Verification items for the finished model (mm, model axes). Coordinates: 2 decimals unless noted, no trailing zeros. Loops run counter-clockwise (first coordinate to the right, second up) from the corner with the lowest first, then second, coordinate; pieces in that order, holes last.
Q1. Sectioned sample at C-C (x = -37.5). Enter the section's corners in (y, z), then the cut area to 3 significant figures.
Q2. Go/stop test with flat-tipped pins: P1, Ø1.9, axis at y = -36, z = 3.5, coming from the -X side; P2, Ø5.5, axis at x = -37.5, y = 0, coming from the +Z side; P3, Ø1.5, axis at x = -16, z = 1.5, coming from the +Y side; P4, Ø3, axis at x = 35, z = 3.5, coming from the -Y side. Record where each tip stops, or that it passes through.
Q3. Sectioned sample at B-B (y = 0). Enter the section's corners in (x, z), then the cut area to 3 significant figures.
Q4. Mould release check, pull along X, two halves, no side actions. Record for faces 1 (the face through (1.47, 49.98, 3.13)), 2 (the face through (-13.675, -34.628, 3.272)), 3 (the face through (-35.302, 0.097, 2.007)): +X half, -X half, draft (parallel to the pull), parting line (faces both ways), or undercut.
Q5. Sectioned sample at D-D (x = -15). Enter the section's corners in (y, z) (3 decimals).
Q6. Material ranges on probe 1 along X at (y, z) = (-20, 1.7); probe 2 along Y at (x, z) = (-5.5, 2); probe 3 along Y at (x, z) = (-1.5, 5.75), recorded low to high.
Q7. Sectioned sample at A-A (x = 0). Enter the section's corners in (y, z).
```python
from build123d import *

# Parameters (mm, degrees)
F0_R           = 50
F1_DEPTH       = 6.35
F3_D           = 4.4
F3_CSINK_D     = 8.96
F3_CSINK_ANGLE = 90
F4_R           = 8
F5_DEPTH       = 8
F7_DEPTH       = 25
F9_R           = 5
F10_D          = 4.4
F11_R          = 7.5
F12_DEPTH      = 25


# Not quite as in the source:
# - a feature names something its author has since deleted; it is built from what else it names


with BuildPart() as f1:
    # F0 (on Top) → F1 (new body)
    with BuildSketch(Plane.XY):
        Circle(F0_R)
    extrude(amount=F1_DEPTH)

    # F3 (through all)
    with Locations(Plane.XY.offset(6.35)):
        with Locations((-37.5, 20), (-37.5, 0), (-37.5, -20), (37.5, 20), (37.5, 0), (37.5, -20)):
            CounterSinkHole(F3_D / 2, F3_CSINK_D / 2, counter_sink_angle=F3_CSINK_ANGLE)

    # F4 (on face) → F5 (cut)
    with BuildSketch(Plane.XY.offset(6.35)):
        Circle(F4_R)
    extrude(amount=-F5_DEPTH, mode=Mode.SUBTRACT)

    # F6 (on face) → F7 (cut)
    with BuildSketch(Plane.XY.offset(6.35)):
        with BuildLine():
            Line((-20, -27.8257569496), (-41.5418734554, -27.8257569496))
            ThreePointArc((-41.5418734554, -27.8257569496), (-32.0601083451, -38.3685998298), (-20, -45.8257569496))
            Line((-20, -45.8257569496), (-20, -27.8257569496))
        make_face()
        with BuildLine():
            ThreePointArc((20, -45.8257569496), (32.0601083451, -38.3685998298), (41.5418734554, -27.8257569496))
            Line((41.5418734554, -27.8257569496), (20, -27.8257569496))
            Line((20, -27.8257569496), (20, -45.8257569496))
        make_face()
    extrude(amount=-F7_DEPTH, mode=Mode.SUBTRACT)

    # F9
    f9_edges = [f1.edges().sort_by_distance(p)[0] for p in [
        (-41.541873, -27.825757, 3.175),
        (-20, -45.825757, 3.175),
        (-20, -27.825757, 3.175),
        (20, -27.825757, 3.175),
        (20, -45.825757, 3.175),
        (41.541873, -27.825757, 3.175),
    ]]
    fillet(f9_edges, radius=F9_R)

    # F10 (through all)
    with Locations(Plane.YZ.offset(20)):
        with Locations((-36.8257569496, 3.175)):
            Hole(F10_D / 2)

    # F11 (on face) → F12 (cut)
    with BuildSketch(Plane.XY.offset(6.35)):
        with Locations((0, -36.8257569496)):
            Circle(F11_R)
    extrude(amount=-F12_DEPTH, mode=Mode.SUBTRACT)


solid = f1.part
```
Geometry check:
1. outline: (-27.83, 0) - (-22.2, 0) - (-22.2, 4.07) - (-24.48, 6.35) - (-27.83, 6.35) - close; (-17.8, 0) - (-2.2, 0) - (-2.2, 4.07) - (-4.48, 6.35) - (-15.52, 6.35) - (-17.8, 4.07) - close; (2.2, 0) - (17.8, 0) - (17.8, 4.07) - (15.52, 6.35) - (4.48, 6.35) - (2.2, 4.07) - close; (22.2, 0) - (33.07, 0) - (33.07, 6.35) - (24.48, 6.35) - (22.2, 4.07) - close
1. area: 287 mm2
2. P1: passes through
2. P2: stops at z = 4.62
2. P3: stops at y = 47.62
2. P4: stops at y = -27.83
3. outline: (-50, 0) - (-39.7, 0) - (-39.7, 4.07) - (-41.98, 6.35) - (-50, 6.35) - close; (-35.3, 0) - (-8, 0) - (-8, 6.35) - (-33.02, 6.35) - (-35.3, 4.07) - close; (8, 0) - (35.3, 0) - (35.3, 4.07) - (33.02, 6.35) - (8, 6.35) - close; (39.7, 0) - (50, 0) - (50, 6.35) - (41.98, 6.35) - (39.7, 4.07) - close
3. area: 467 mm2
4. face 1: parting line
4. face 2: draft
4. face 3: undercut
5. outline: (-47.697, 0) - (47.697, 0) - (47.697, 6.35) - (-47.697, 6.35) - close; hole circle Ø4.4 at (-36.826, 3.175)
6. probe 1: x = -45.83 to -39.7, -35.3 to 35.3, 39.7 to 45.83
6. probe 2: y = -49.7 to -41.92, -31.73 to -5.81, 5.81 to 49.7
6. probe 3: y = -49.98 to -44.17, -29.48 to -7.86, 7.86 to 49.98
7. outline: (-50, 0) - (-44.33, 0) - (-44.33, 6.35) - (-50, 6.35) - close; (-29.33, 0) - (-8, 0) - (-8, 6.35) - (-29.33, 6.35) - close; (8, 0) - (50, 0) - (50, 6.35) - (8, 6.35) - close
